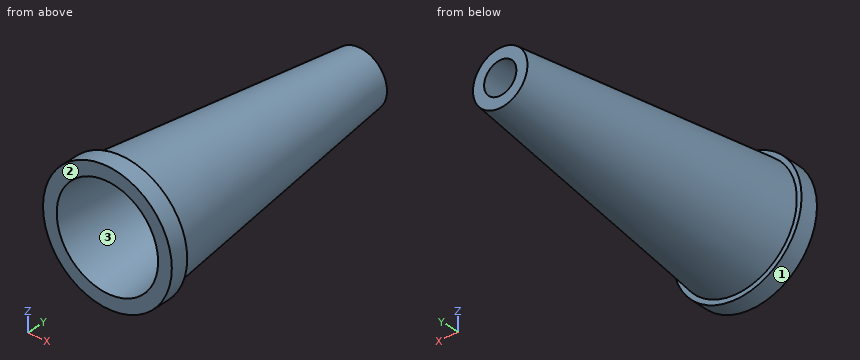
from build123d import *

# Parameters (mm, degrees)
F0_R     = 4.2672
F2_R     = 1.8796
F4_T     = -0.762
F5_R     = 4.445
F5_R_2   = 3.4997563168
F6_DEPTH = 1.2192


with BuildPart() as f3:
    # F0 (on Front) → F3 section 0
    with BuildSketch(Plane.XZ):
        Circle(F0_R)
    # F2 (on offset) → F3 section 1
    with BuildSketch(Plane.XZ.offset(-19.939)):
        Circle(F2_R)
    loft()

    # F4
    f4_openings = [f3.faces().sort_by_distance(p)[0] for p in [
        (0, 0, 0),
        (0, 19.939, 0),
    ]]
    offset(amount=F4_T, openings=f4_openings, kind=Kind.INTERSECTION)

    # F5 (on Front) → F6 (join)
    with BuildSketch(Plane.XZ):
        Circle(F5_R)
        Circle(F5_R_2, mode=Mode.SUBTRACT)
    extrude(amount=-F6_DEPTH)


solid = f3.part
The listing builds one solid part. Answer for the finished solid, in the listing's coordinates (mm). Face numbers are marked on the shaded views. Give positions to 0.01 mm unless a question says otherwise; leave off trailing zeros. Write each loop counter-clockwise with the first axis right and the second up, starting at its lowest first coordinate (ties: lowest second). Pieces come first, ordered by that corner, then holes. Notation, with made-up numbers: (74.5, -39.5) -> (115.5, -39.5) arc R32 cw to (115.5, -8.5) -> close; hole circle Ø11 at (-31.5, 63). An arc over 180 degrees is marked (long way). Use a Markdown table: item, result.
(1) Determine the mould class of the marked faces 1, 2 and 3 for opening direction Z: released by +Z, released by -Z, zero draft, split by the parting line, or undercut.
Return value:
| item | result |
|---|---|
| face 1 | split by the parting line |
| face 2 | zero draft |
| face 3 | undercut |
(2) Section A-A, the plane x = 0 is taken. Determine the outline of the cut face in (y, z) (3 decimals), then the cut area to 3 significant figures.
Return value:
| item | result |
|---|---|
| outline | (0, -4.445) -> (1.219, -4.445) -> (1.219, -4.121) -> (19.939, -1.88) -> (19.939, -1.112) -> (0, -3.5) -> close; (0, 3.5) -> (19.939, 1.112) -> (19.939, 1.88) -> (1.219, 4.121) -> (1.219, 4.445) -> (0, 4.445) -> close |
| area | 31.2 mm2 |
(3) Flat-ended cylindrical pins translate along their axes: P1, Ø1.5, axis at x = 0.5, y = 2, coming from the -Z side; P2, Ø2, axis at y = 5, z = 3, coming from the -X side; P3, Ø5, axis at y = 13.5, z = -1, coming from the -X side. Find the tip coordinate at first contact, or state that the pin passes through.
Return value:
| item | result |
|---|---|
| P1 | z = -4.11 |
| P2 | x = -3.09 |
| P3 | x = -2.93 |
(4) Find the intervals of material crossed by probe 1 along X at (y, z) = (1, 1); probe 2 along X at (y, z) = (11.5, 0.25); probe 3 along Z at (x, y) = (-2.5, 6.5), in increasing order. Write a range as from..to.
Return value:
| item | result |
|---|---|
| probe 1 | -4.33..-3.23, 3.23..4.33 |
| probe 2 | -2.88..-2.11, 2.11..2.88 |
| probe 3 | -2.43..-1.08, 1.08..2.43 |
(5) Section C-C, the plane y = 16 is taken. Determine the outline of the cut face in (x, z), then the cut area to 3 significant figures.
Return value:
| item | result |
|---|---|
| outline | circle Ø4.7 at (0, 0); hole circle Ø3.17 at (0, 0) |
| area | 9.49 mm2 |
(6) Section B-B, the plane y = 11.25 is taken. Determine the outline of the cut face in (x, z), then the cut area to 3 significant figures.
Return value:
| item | result |
|---|---|
| outline | circle Ø5.84 at (0, 0); hole circle Ø4.31 at (0, 0) |
| area | 12.2 mm2 |
